The listing builds one solid part. Answer for the finished solid, in the listing's coordinates (mm). A direction names the side the tool comes from. Give positions to 0.01 mm unless a question says otherwise; leave off trailing zeros. Write each loop counter-clockwise with the first axis right and the second up, starting at its lowest first coordinate (ties: lowest second). Pieces come first, ordered by that corner, then holes. Notation, with made-up numbers: (9.25, 88) -> (56.25, 88) arc R20 ccw to (56.25, 120) -> close; hole circle Ø6 at (-6, 21). An arc over 180 degrees is marked (long way). Put each result on its own line as item: value. Start each with the question number.
1) A cutting plane is placed at D-D (z = -16.5). Write down the section's boundary in (x, y).
2) Find the intervals of material crossed by line 1 along Z through (x, y) = (12, -0.5); line 2 along X through (y, z) = (3.25, -6.25); line 3 along Y through (x, z) = (0, -29.25), in increasing order. Write a range as from..to.
3) For faces 1 (the flat face through (-15.997, 1, -15)), 2 (the flat face through (0, -5, -2)), 3 (the cylindrical face through (-1.63, -7.34, -29.11)), determine the directions among +Z, -Z, +X, -X, +Y, -Y from which every point of the face is accessible in a straight line to the end or side of a thin tool.
4) A cutting plane is placed at B-B (z = -7). Write down the section's boundary in (x, y).
5) For a pull along X with two mould halves and no side action, classify faces 4 (the cylindrical face through (-1.63, -7.34, -0.89)), 5 (the flat face through (16.524, -4.549, -14.79)), 6 (the flat face through (12, -10.974, -15)), 7 (the flat face through (-17.03, -8, -15)) as released by +X, released by -X, zero draft, split by the parting line, or undercut.
6) Flat-ended cylindrical pins translate along their axes: pin 1 Ø3.5 at (x, z) = (12, -9.5) entering from +Y; pin 2 Ø12 at (y, z) = (2.5, -11) entering from +X; pin 3 Ø7 at (x, y) = (2.5, -1) entering from +Z. Find the tip coordinate at first contact, or state that the pin passes through.
7) A cutting plane is placed at A-A (x = 12). Write down the section's boundary in (y, z), then the cut area to 3 significant figures.
from build123d import *

# Parameters (mm, degrees)
ESQUISSE1_R             = 7.519017315
BOSS_EXTRU_1_DEPTH      = 30
ESQUISSE1_3_R           = 7.051788316
ESQUISSE1_3_R_2         = 4.523392982
BOSS_EXTRU_2_DEPTH      = 28
ESQUISSE1_4_R           = 7.519017315
ESQUISSE1_4_R_2         = 7.051788316
BOSS_EXTRU_3_DEPTH      = 30
ESQUISSE1_5_R           = 4.523392982
ESQUISSE1_5_R_2         = 4
BOSS_EXTRU_4_DEPTH      = 28.5
ESQUISSE1_6_R           = 4.523392982
ESQUISSE1_6_R_2         = 4
ENL_V_MAT_EXTRU_1_DEPTH = 1.5
ESQUISSE1_7_R           = 7.051788316
ESQUISSE1_7_R_2         = 4.523392982
ENL_V_MAT_EXTRU_2_DEPTH = 2
ESQUISSE1_8_R           = 7.519017315
ESQUISSE1_8_R_2         = 7.051788316
ENL_V_MAT_EXTRU_3_DEPTH = 1.8
ENL_V_START             = -30
ESQUISSE1_9_R           = 7.519017315
ESQUISSE1_9_R_2         = 7.051788316
ENL_V_MAT_EXTRU_4_DEPTH = 1.8
ESQUISSE2_R             = 1.65
ENL_V_MAT_EXTRU_5_DEPTH = 21.8


with BuildPart() as part:
    # Esquisse1 → Boss.-Extru.1 (new body)
    with BuildSketch(Plane.XY):
        Polygon((-15.997216081, -4.089203195), (-17.03, -5.004453984), (-17.03, -10.973805396), (-7.66267479, -10.973805396), (-7.153229177, -10.464359784), (6.857616233, -10.464359784), (7.367061846, -10.973805396), (17.03, -10.973805396), (17.03, -4.995255883), (16.002783919, -4.089203195), (16.002783919, 6.07141612), (15.037454618, 6.944265115), (8.081929489, 6.944265115), (4, 11.026194604), (-4, 11.026194604), (-8.083891517, 6.944265115), (-15.124367087, 6.944265115), (-15.997216081, 6.07141612), align=None)
        Circle(ESQUISSE1_R, mode=Mode.SUBTRACT)
    extrude(amount=-BOSS_EXTRU_1_DEPTH)



with BuildPart() as body_2:
    # Esquisse1_3 → Boss.-Extru.2 (new body)
    with BuildSketch(Plane.XY):
        Circle(ESQUISSE1_3_R)
        Circle(ESQUISSE1_3_R_2, mode=Mode.SUBTRACT)
    extrude(amount=-BOSS_EXTRU_2_DEPTH)


with BuildPart() as part_1:
    add(part.part)

    add(body_2.part)  # Boss.-Extru.3 merges body 2
    # Esquisse1_4 → Boss.-Extru.3 (add)
    with BuildSketch(Plane.XY):
        Circle(ESQUISSE1_4_R)
        Circle(ESQUISSE1_4_R_2, mode=Mode.SUBTRACT)
    extrude(amount=-BOSS_EXTRU_3_DEPTH)

    # Esquisse1_5 → Boss.-Extru.4 (add)
    with BuildSketch(Plane.XY):
        Circle(ESQUISSE1_5_R)
        Circle(ESQUISSE1_5_R_2, mode=Mode.SUBTRACT)
    extrude(amount=-BOSS_EXTRU_4_DEPTH)

    # Esquisse1_6 → Enl_v. mat.-Extru.1 (cut)
    with BuildSketch(Plane.XY):
        Circle(ESQUISSE1_6_R)
        Circle(ESQUISSE1_6_R_2, mode=Mode.SUBTRACT)
    extrude(amount=-ENL_V_MAT_EXTRU_1_DEPTH, mode=Mode.SUBTRACT)

    # Esquisse1_7 → Enl_v. mat.-Extru.2 (cut)
    with BuildSketch(Plane.XY):
        Circle(ESQUISSE1_7_R)
        Circle(ESQUISSE1_7_R_2, mode=Mode.SUBTRACT)
    extrude(amount=-ENL_V_MAT_EXTRU_2_DEPTH, mode=Mode.SUBTRACT)

    # Esquisse1_8 → Enl_v. mat.-Extru.3 (cut)
    with BuildSketch(Plane.XY):
        Circle(ESQUISSE1_8_R)
        Circle(ESQUISSE1_8_R_2, mode=Mode.SUBTRACT)
    extrude(amount=-ENL_V_MAT_EXTRU_3_DEPTH, mode=Mode.SUBTRACT)

    # Esquisse1_9 → Enl_v. mat.-Extru.4 (cut)
    with BuildSketch(Plane.XY.offset(ENL_V_START)):
        Circle(ESQUISSE1_9_R)
        Circle(ESQUISSE1_9_R_2, mode=Mode.SUBTRACT)
    extrude(amount=ENL_V_MAT_EXTRU_4_DEPTH, mode=Mode.SUBTRACT)

    # Esquisse2 → Enl_v. mat.-Extru.5 (cut)
    with BuildSketch(Plane.XZ.offset(10.973805396)):
        with Locations((-12, -7)):
            Circle(ESQUISSE2_R)
        with Locations((12, -7)):
            Circle(ESQUISSE2_R)
        with Locations((12, -23)):
            Circle(ESQUISSE2_R)
        with Locations((-12, -23)):
            Circle(ESQUISSE2_R)
    extrude(amount=-ENL_V_MAT_EXTRU_5_DEPTH, mode=Mode.SUBTRACT)


solid = part_1.part
Reply:
1. outline: (-17.03, -10.97) -> (-7.66, -10.97) -> (-7.15, -10.46) -> (6.86, -10.46) -> (7.37, -10.97) -> (17.03, -10.97) -> (17.03, -5) -> (16, -4.09) -> (16, 6.07) -> (15.04, 6.94) -> (8.08, 6.94) -> (4, 11.03) -> (-4, 11.03) -> (-8.08, 6.94) -> (-15.12, 6.94) -> (-16, 6.07) -> (-16, -4.09) -> (-17.03, -5) -> close; hole circle Ø8 at (0, 0)
2. line 1: z = -30..-24.65, -21.35..-8.65, -5.35..0
2. line 2: x = -16..-13.47, -10.53..-2.33, 2.33..10.53, 13.47..16
2. line 3: y = -10.46..-7.52, 7.52..11.03
3. face 1: +Z, -Z, -X, +Y
3. face 2: +Z
3. face 3: -Z
4. outline: (-17.03, -10.97) -> (-13.65, -10.97) -> (-13.65, 6.94) -> (-15.12, 6.94) -> (-16, 6.07) -> (-16, -4.09) -> (-17.03, -5) -> close; (-10.35, -10.97) -> (-7.66, -10.97) -> (-7.15, -10.46) -> (6.86, -10.46) -> (7.37, -10.97) -> (10.35, -10.97) -> (10.35, 6.94) -> (8.08, 6.94) -> (4, 11.03) -> (-4, 11.03) -> (-8.08, 6.94) -> (-10.35, 6.94) -> close; (13.65, -10.97) -> (17.03, -10.97) -> (17.03, -5) -> (16, -4.09) -> (16, 6.07) -> (15.04, 6.94) -> (13.65, 6.94) -> close; hole circle Ø8 at (0, 0)
5. face 4: undercut
5. face 5: released by +X
5. face 6: zero draft
5. face 7: released by -X
6. pin 1: stops at y = 6.94
6. pin 2: stops at x = 16
6. pin 3: stops at z = -1.5
7. outline: (-10.97, -30) -> (6.94, -30) -> (6.94, -24.65) -> (-10.97, -24.65) -> close; (-10.97, -21.35) -> (6.94, -21.35) -> (6.94, -8.65) -> (-10.97, -8.65) -> close; (-10.97, -5.35) -> (6.94, -5.35) -> (6.94, 0) -> (-10.97, 0) -> close
7. area: 419 mm2
